```python
from build123d import *

# Parameters (mm, degrees)
SKETCH1_W           = 20
SKETCH1_H           = 10
SKETCH1_R           = 1.25
BOSS_EXTRUDE1_DEPTH = 6
SKETCH2_R           = 0.75
BOSS_EXTRUDE2_DEPTH = 1


with BuildPart() as part:
    # Sketch1 → Boss-Extrude1 (new body)
    with BuildSketch(Plane.XY):
        Rectangle(SKETCH1_W, SKETCH1_H)
        with Locations((-5, -2.5)):
            Circle(SKETCH1_R, mode=Mode.SUBTRACT)
        with Locations((5, -2.5)):
            Circle(SKETCH1_R, mode=Mode.SUBTRACT)
    extrude(amount=BOSS_EXTRUDE1_DEPTH)

    # Sketch2 → Boss-Extrude2 (add)
    with BuildSketch(Plane(origin=(0, 5, 0), x_dir=(1, 0, 0), z_dir=(0, 1, 0))):
        with Locations((3, -3)):
            Circle(SKETCH2_R)
    extrude(amount=BOSS_EXTRUDE2_DEPTH)


solid = part.part
```
Read the model definition and answer for the solid it produces. Units are mm, in the model's axes. A direction names the side the tool comes from. Coordinates: 2 decimals unless noted, no trailing zeros. Write each loop counter-clockwise with the first axis right and the second up, starting at its lowest first coordinate (ties: lowest second). Pieces come first, ordered by that corner, then holes. Notation, with made-up numbers: (-19, 29) - (25, 29) arc R16 ccw to (25, 35) - close; hole circle Ø1 at (26.5, 50.5). An arc over 180 degrees is marked (long way). Answer as a JSON object with one key per item and string values. Group by question number.
1. The mould has two halves that part along Y. Classify faces 3 (the flat face through (0, 5, 3)), 4 (the flat face through (10, 0, 3)), 5 (the cylindrical face through (-6.25, -2.45, 2.96)): +Y half, -Y half, draft (parallel to the pull), parting line (faces both ways), or undercut.
2. A cutting plane is placed at B-B (y = -2.5). Determine the outline of the cut face in (x, z).
3. Consider L1, parallel to Y at x = 5, z = 1.5; L2, parallel to X at y = -2.75, z = 5; L3, parallel to X at y = -1.5, z = 4.3. Determine where each line is inside the solid, lowest interval first. Write a range as [from, to].
4. Which of the six approach directions +Z, -Z, +X, -X, +Y, -Y give full straight-line access (tool end or side, diameter ignored) to faces 1 (the cylindrical face through (2.405, 5.493, 3.456)), 2 (the flat face through (0, 0, 6))?
5. A cutting plane is placed at C-C (z = 5.2). Determine the outline of the cut face in (x, y).
6. A cutting plane is placed at A-A (x = -5). Determine the outline of the cut face in (y, z), plus the area to 3 significant figures.
7. A cutting plane is placed at D-D (x = 5.75). Determine the outline of the cut face in (y, z), plus the area to 3 significant figures.
8. This flat-tipped pin is pushed along its axis until it touches: P1, Ø1.5, axis at x = -1, z = 5.5, coming from the +Y side. Where does it stop, or does it pass through?
Worked out:
{
 "1": {"face 3": "+Y half", "face 4": "draft", "face 5": "undercut"},
 "2": {"outline": "(-10, 0) - (-6.25, 0) - (-6.25, 6) - (-10, 6) - close; (-3.75, 0) - (3.75, 0) - (3.75, 6) - (-3.75, 6) - close; (6.25, 0) - (10, 0) - (10, 6) - (6.25, 6) - close"},
 "3": {"L1": "y = [-5, -3.75], [-1.25, 5]", "L2": "x = [-10, -6.22], [-3.78, 3.78], [6.22, 10]", "L3": "x = [-10, -5.75], [-4.25, 4.25], [5.75, 10]"},
 "4": {"face 1": "+Y", "face 2": "+Z, +X, -X, +Y, -Y"},
 "5": {"outline": "(-10, -5) - (10, -5) - (10, 5) - (-10, 5) - close; hole circle Ø2.5 at (-5, -2.5); hole circle Ø2.5 at (5, -2.5)"},
 "6": {"outline": "(-5, 0) - (-3.75, 0) - (-3.75, 6) - (-5, 6) - close; (-1.25, 0) - (5, 0) - (5, 6) - (-1.25, 6) - close", "area": "45.0 mm²"},
 "7": {"outline": "(-5, 0) - (-3.5, 0) - (-3.5, 6) - (-5, 6) - close; (-1.5, 0) - (5, 0) - (5, 6) - (-1.5, 6) - close", "area": "48.0 mm²"},
 "8": {"P1": "stops at y = 5"}
}
